Here's how the part is built. I have some questions about the finished solid (model axes, mm). A direction names the side the tool comes from. Round coordinates to 2 decimals unless told otherwise and drop trailing zeros. Order: outer loops, then holes, each group sorted by start corner. A loop starts at its lowest first (then second) coordinate and runs counter-clockwise, first axis right, second up.
```python
from build123d import *

# Parameters (mm, degrees)
EXTRUDE_1_DEPTH  = 88
CHAMFER_1_SIZE   = 13
CHAMFER_1_SIZE2  = 22.516660498
CHAMFER_2_SIZE   = 4.330127019
CHAMFER_2_SIZE_2 = 2.5


with BuildPart() as part:
    # Эскиз1 → Бобышка-Вытянуть1 (new body)
    with BuildSketch(Plane.XY.offset(1548)):
        Polygon((36.549287829, 66.569518917), (29.833037542, 66.569518917), (29.833037542, 81.891176087), (39.628851143, 81.891176087), (40.549825071, 82.812150015), (40.549825071, 85.491346897), (39.21022663, 84.151748456), (37.368278773, 84.151748456), (37.368278773, 85.491346897), (40.549825071, 89.761316928), (40.549825071, 94.198736764), (39.628851143, 92.962692808), (39.628851143, 91.017190466), (36.549287829, 91.017190466), (36.549287829, 92.962692808), (45.40586942, 103.324751144), (45.40586942, 103.910825462), (43.982546076, 103.910825462), (41.660685836, 100.794644613), (40.977578624, 100.794644613), (40.977578624, 101.303626458), (43.620510787, 104.850719623), (50.100205342, 105.797191861), (64.411422303, 105.797191861), (66.943124576, 103.910825462), (66.943124576, 101.303626458), (46.860358064, 101.303626458), (44.694207748, 100.794644613), (44.694207748, 78.667767338), (36.549287829, 78.667767338), align=None)
    extrude(amount=EXTRUDE_1_DEPTH)

    # Фаска1
    chamfer_1_edges = [part.edges().sort_by_distance(p)[0] for p in [
        (66.943124576, 102.60722596, 1548),
    ]]
    chamfer_1_side = [part.faces().sort_by_distance(p)[0] for p in [
        (43.066294454, 88.644441119, 1548),
    ]]
    chamfer(chamfer_1_edges, length=CHAMFER_1_SIZE, length2=CHAMFER_1_SIZE2, reference=chamfer_1_side[0])

    # Фаска2
    # the kernel refuses this chamfer: 4.330127019, 2.5 mm, written as the material it takes off along each edge
    with BuildSketch(Plane(origin=(40.977578624, 89.592234687, 1636), x_dir=(0.9998132206222081, 0, 0.01932676561269257), z_dir=(0, 1, 0))) as chamfer_2_piece_1_section:
        Polygon((CHAMFER_2_SIZE * 0.999813220604, CHAMFER_2_SIZE * 0.0193267656123), (-CHAMFER_2_SIZE_2 * 0.0193267656127, CHAMFER_2_SIZE_2 * 0.999813220622), (0, 0), align=None)
    chamfer_2_piece_1 = extrude(amount=22.913801697, mode=Mode.PRIVATE)
    chamfer_2_piece_1 = split(chamfer_2_piece_1, bisect_by=Plane(origin=(45.427089539, 103.349578342, 1635.744871049), z_dir=(-0.7601686994393885, 0.6497257485990753, 0)), keep=Keep.TOP, mode=Mode.PRIVATE)
    add(chamfer_2_piece_1, mode=Mode.SUBTRACT)


solid = part.part
```
1) We'd pull the mould along X, two halves only. Please class faces 6 (the flat face through (29.833, 74, 1591)), 7 (the flat face through (43, 88, 1636)), 8 (the flat face through (40.55, 92, 1591)): +X half, -X half, draft (parallel to the pull), parting line (faces both ways), or undercut.
2) For faces 1 (the flat face through (35, 81.891, 1591)), 2 (the flat face through (42.838, 102.375, 1591.007)), 3 (the flat face through (41, 78.668, 1591)), 4 (the flat face through (43.153, 103.095, 1634.756)), 5 (the flat face through (36.549, 92, 1591)), which set-ups out of +Z, -Z, +X, -X, +Y, -Y let a thin tool reach every point of the face, with its end or its side?
3) If we section it at C-C (y = 77): Write out the boundary of the cut face in (x, z).
4) I need wall thicknesses on line 1 (Y direction, x = 39, z = 1613.5); line 2 (Y direction, x = 62, z = 1583); line 3 (X direction, y = 80.5, z = 1578). Which ranges of each line are inside material? Lowest first, please.
5) I'm going to push flat-ended pins straight in: pin 1 (0.6 mm diameter, centred on y = 92, z = 1575, fed in from +X); pin 2 (1.6 mm diameter, centred on x = 45, z = 1608.5, fed in from -Y); pin 3 (6 mm diameter, centred on y = 88.5, z = 1598.5, fed in from -X). Where does each tip first touch, or does it pass through?
6) If we section it at B-B (x = 34): Write out the boundary of the cut face in (y, z).
Solutions:
1. face 6: -X half
1. face 7: draft
1. face 8: undercut
2. face 1: +Z, -Z, -X
2. face 2: +Z, -Z
2. face 3: +Z, -Z, +X, -Y
2. face 4: +Z, -X, +Y
2. face 5: +Z, -Z, -X, +Y
3. outline: (29.83, 1548) - (36.55, 1548) - (36.55, 1636) - (29.83, 1636) - close
4. line 1: y = 78.67 to 81.89, 84.15 to 87.68, 91.02 to 95.83
4. line 2: y = 101.3 to 105.8
4. line 3: x = 29.83 to 44.69
5. pin 1: stops at x = 44.69
5. pin 2: stops at y = 78.67
5. pin 3: stops at x = 36.55
6. outline: (66.57, 1548) - (81.89, 1548) - (81.89, 1636) - (66.57, 1636) - close
